The model under review builds one solid part; all positions refer to its coordinate system, in mm. Round coordinates to 2 decimals unless told otherwise and drop trailing zeros. Loops run counter-clockwise (first coordinate to the right, second up) from the corner with the lowest first, then second, coordinate; pieces in that order, holes last. Notation, with made-up numbers: M 53,76 L 112,76 A26 cw 112,93 Z; hole C 14.25,38.5 d6. An arc over 180 degrees is marked long. Use a Markdown table: item, result. Add a question column.
Autodesk Inventor part; units mm, degrees
ref_plane "YZ Plane" through (0, 0, 0) normal (1, 0, 0) x (0, 1, 0)
ref_plane "XZ Plane" through (0, 0, 0) normal (0, 1, 0) x (-1, 0, 0)
ref_plane "XY Plane" through (0, 0, 0) normal (0, 0, 1) x (1, 0, 0)
sketch "Sketch1" plane through (0, 0, 0) normal (1, 0, 0) x (0, 1, 0)
  line L0 (15.875, 6.35) -> (-15.875, 6.35)
  line L1 (-15.875, 6.35) -> (-15.875, -6.35)
  line L2 (-15.875, -6.35) -> (15.875, -6.35)
  line L3 (15.875, -6.35) -> (15.875, 6.35)
  line L4 (15.875, 6.35) -> (-15.875, -6.35) construction
  line L5 (-15.875, 6.35) -> (15.875, -6.35) construction
  point P0 (0, 0)
  dimension "d0" = 31.75
  dimension "d1" = 12.7
extrude "Extrusion1" add sketch "Sketch1" along normal blind 12.7
sketch "Sketch2" plane through (12.7, 0, 0) normal (1, 0, 0) x (0, 0, -1)
  line L0 (6.35, 15.875) -> (-6.35, 15.875)
  point P0 (0, 0)
  point P1 (0, -9.525)
  point P2 (0, 3.175)
  dimension "d4" = 12.7
  dimension "d5" = 12.7
hole "Hole1" at (12.7, -9.525, 0) at (12.7, 3.175, 0) direction (-1, 0, 0) diameter 6.096 depth 25.4 tip angle 118
sketch "Sketch3" plane through (0, -15.875, 6.35) normal (0, 0, 1) x (1, 0, 0)
  line L0 (0, 31.75) -> (12.7, 31.75)
  point P0 (0, 15.875)
  point P1 (6.35, 25.4)
  point P2 (6.35, 12.7)
  point P3 (6.35, 31.75)
  dimension "d13" = 12.7
  dimension "d14" = 6.35
hole "Hole2" at (6.35, 9.525, 6.35) at (6.35, -3.175, 6.35) direction (0, 0, -1) diameter 6.096 depth 25.4 tip angle 118
fillet "Fillet1" radius 1.5875 4 edges at (12.7, -15.875, 0) (0, -15.875, 0) (12.7, 15.875, 0) (0, 15.875, 0)
properties part number "3DPRINT,NUT-BLOCK" material "Nylon 6/6"
(1) Consider section B-B, the plane x = 4. Give the boundary of the cut face in (y, z) (3 decimals).
(2) Insertion check: pin 1 Ø5 at (y, z) = (10, 1.5) entering from -X; pin 2 Ø5.5 at (x, y) = (6.35, 9.525) entering from +Z. Each pin has a flat end and moves straight along its axis. Give the tip position at first contact, or say it passes through.
(3) To check wall thickness, follow probe 1 along Y at (x, z) = (6.35, -3.5) (3 decimals); probe 2 along Y at (x, z) = (5.75, 5.5) (3 decimals); probe 3 along Y at (x, z) = (6, 0.75) (3 decimals). State the ranges of each line that lie inside material, in increasing order.
(4) Consider section A-A, the plane z = 0. Give the number of separate pieces and of enclosed holes in the cut face, then the cut area to 3 significant figures.
(5) Draft analysis for pull direction X (two halves, no side actions). For faces 1 (the face through (6.22, 12.57, -0.09)), 2 (the face through (12.247, -15.398, -0.089)), 3 (the face through (0.477, 15.422, 0.089)), 4 (the face through (6.26, -6.55, 0.66)), state which applies: released by +X, released by -X, zero draft, split by the parting line, or undercut.
(6) Consider section C-C, the plane y = 9.5. Give the boundary of the cut face in (x, z), then the cut area to 3 significant figures.
Found:
| question | item | result |
|---|---|---|
| 1 | outline | M -15.875,-6.35 L -5.116,-6.35 L -5.116,6.35 L -15.875,6.35 Z; M -1.234,-6.35 L 7.584,-6.35 L 7.584,6.35 L -1.234,6.35 Z; M 11.466,-6.35 L 15.875,-6.35 L 15.875,6.35 L 11.466,6.35 Z; hole C -9.525,0 d6.096; hole C 3.175,0 d6.096 |
| 2 | pin 1 | stops at x = 0 |
| 2 | pin 2 | passes through |
| 3 | probe 1 | y = -15.875 to -6.223, -0.127 to 6.477, 12.573 to 15.875 |
| 3 | probe 2 | y = -15.875 to -6.163, -0.187 to 6.537, 12.513 to 15.875 |
| 3 | probe 3 | y = -15.875 to -12.479, -6.571 to -6.203, -0.147 to 0.221, 6.129 to 6.497, 12.553 to 15.875 |
| 4 | separate pieces | 3 |
| 4 | enclosed holes | 2 |
| 4 | area | 188 mm^2 |
| 5 | face 1 | undercut |
| 5 | face 2 | released by +X |
| 5 | face 3 | released by -X |
| 5 | face 4 | zero draft |
| 6 | outline | M 0,-6.35 L 3.3,-6.35 L 3.3,6.35 L 0,6.35 Z; M 9.4,-6.35 L 12.7,-6.35 L 12.7,6.35 L 9.4,6.35 Z |
| 6 | area | 83.9 mm^2 |
